```python
from build123d import *

# Parameters (mm, degrees)
CYLINDER001_R     = 5
CYLINDER001_DEPTH = 10
CYLINDER_R        = 5
CYLINDER_DEPTH    = 10
BOX001_W          = 30
BOX001_H          = 15
BOX001_DEPTH      = 10
BOX_W             = 70
BOX_H             = 40
BOX_DEPTH         = 4


with BuildPart() as cylinder001:
    # Cylinder001 → Cylinder001 (new body)
    with BuildSketch(Plane(origin=(60, 30, 0), x_dir=(1, 0, 0), z_dir=(0, 0, 1))):
        Circle(CYLINDER001_R)
    extrude(amount=CYLINDER001_DEPTH)


with BuildPart() as cylinder:
    # Cylinder → Cylinder (new body)
    with BuildSketch(Plane(origin=(10, 30, 0), x_dir=(1, 0, 0), z_dir=(0, 0, 1))):
        Circle(CYLINDER_R)
    extrude(amount=CYLINDER_DEPTH)


with BuildPart() as cube001:
    # Box001 → Box001 (new body)
    with BuildSketch(Plane(origin=(20, 25, 0), x_dir=(1, 0, 0), z_dir=(0, 0, 1))):
        with Locations((15, 7.5)):
            Rectangle(BOX001_W, BOX001_H)
    extrude(amount=BOX001_DEPTH)


with BuildPart() as cut002:
    # Box → Box (new body)
    with BuildSketch(Plane.XY):
        with Locations((35, 20)):
            Rectangle(BOX_W, BOX_H)
    extrude(amount=BOX_DEPTH)

    # Cut: cut Cube001
    add(cube001.part, mode=Mode.SUBTRACT)

    # Cut001: cut Cylinder
    add(cylinder.part, mode=Mode.SUBTRACT)

    # Cut002: cut Cylinder001
    add(cylinder001.part, mode=Mode.SUBTRACT)


solid = cut002.part
```
Input: part model. Units: mm. Frame: model coordinates. A direction names the side the tool comes from. Coordinates: 2 decimals unless noted, no trailing zeros. Loops run counter-clockwise (first coordinate to the right, second up) from the corner with the lowest first, then second, coordinate; pieces in that order, holes last. Notation, with made-up numbers: M 40.5,45 L 61.5,45 A14 ccw 61.5,64 Z; hole C 6.5,6.5 d2. An arc over 180 degrees is marked long. One line per item, written item: value.
(1) Section A-A (z = 1.65). Output: boundary loops of the cut face in (x, y), and give its area (3 significant figures).
Filled in:
outline: M 0,0 L 70,0 L 70,40 L 50,40 L 50,25 L 20,25 L 20,40 L 0,40 Z; hole C 10,30 d10; hole C 60,30 d10
area: 2,190 mm^2
(2) Line query: line 1 along X through (y, z) = (30, 1.5); line 2 along Y through (x, z) = (10, 2); line 3 along X through (y, z) = (26, 1.25). Output: solid intervals per line, ascending. Write a range as from..to.
Filled in:
line 1: 0..5, 15..20, 50..55, 65..70
line 2: 0..25, 35..40
line 3: 0..7, 13..20, 50..57, 63..70
(3) Pin query (flat end, axial travel): pin 1 (2 mm diameter, centred on x = 24.5, z = 3.5, fed in from +Y); pin 2 (9 mm diameter, centred on x = 10, y = 30, fed in from +Z). Return the tip coordinate at first contact, or that it passes through.
Filled in:
pin 1: y = 25
pin 2: through
(4) Section C-C (y = 30). Output: boundary loops of the cut face in (x, z), and give its area (3 significant figures).
Filled in:
outline: M 0,0 L 5,0 L 5,4 L 0,4 Z; M 15,0 L 20,0 L 20,4 L 15,4 Z; M 50,0 L 55,0 L 55,4 L 50,4 Z; M 65,0 L 70,0 L 70,4 L 65,4 Z
area: 80.0 mm^2
(5) Reachability of faces 4 (the flat face through (35, 0, 2)), 5 (the flat face through (35, 25, 2)) from +Z, -Z, +X, -X, +Y, -Y: full face, straight path, thin tool, end or side. Return the list, or none.
Filled in:
face 4: +Z, -Z, +X, -X, -Y
face 5: +Z, -Z, +Y
(6) Section D-D (x = 41). Output: boundary loops of the cut face in (y, z), and give its area (3 significant figures).
Filled in:
outline: M 0,0 L 25,0 L 25,4 L 0,4 Z
area: 100 mm^2
(7) Section B-B (x = 14). Output: boundary loops of the cut face in (y, z).
Filled in:
outline: M 0,0 L 27,0 L 27,4 L 0,4 Z; M 33,0 L 40,0 L 40,4 L 33,4 Z
(8) Pull-direction query (X, two-part tool) for faces 1 (the flat face through (35, 16, 4)), 2 (the flat face through (70, 20, 2)), 3 (the flat face through (20, 32, 2)); classes: +X half, -X half, draft (parallel to the pull), parting line (faces both ways), or undercut.
Filled in:
face 1: draft
face 2: +X half
face 3: undercut
